Work out the finished part from the listing and answer in its coordinate system (mm). A direction names the side the tool comes from. Round coordinates to 2 decimals unless told otherwise and drop trailing zeros. Write each loop counter-clockwise with the first axis right and the second up, starting at its lowest first coordinate (ties: lowest second). Pieces come first, ordered by that corner, then holes. Notation, with made-up numbers: M 85,2 L 144,2 A14 ccw 144,14 Z; hole C 34.5,63.25 d4. An arc over 180 degrees is marked long. One line per item, written item: value. Start each with the question number.
Q1. A tool of negligible diameter and unlimited length cuts with its end or side. For faces 1 (the flat face through (19.2, -4.8, -2)), 2 (the flat face through (-0.29, -8, 2)), 3 (the flat face through (29.71, -7, 2)), 4 (the flat face through (15, 0, 2)), 5 (the flat face through (15, -15, 2)), from which of +Z, -Z, +X, -X, +Y, -Y can it reach the whole face along a straight path? Write none if from no direction.
Q2. Find section D-D (y = 1.25). Write down the section's boundary in (x, z).
Q3. Find section A-A (y = -7.5). Write down the section's boundary in (x, z).
Q4. Consider probe 1 along Z at (x, y) = (27.5, -16.5); probe 2 along Z at (x, y) = (13, -14); probe 3 along X at (y, z) = (-9.25, -13.5). Determine where each line is inside the solid, lowest interval first.
Q5. Find section B-B (x = 3.5). Write down the section's boundary in (y, z).
Q6. Given pin 1 Ø10 at (x, z) = (7, -12) entering from -Y; pin 2 Ø1 at (x, z) = (19.5, 2) entering from +Y; pin 3 Ø2 at (y, z) = (-7.5, -12) entering from -X; pin 4 Ø10 at (y, z) = (-3, 0.5) entering from +X, each flat-ended and moving along its own axis, determine where each tip first touches the part or whether it passes through.
Q7. Find section C-C (z = -7.25). Write down the section's boundary in (x, y), and give its area (3 significant figures).
Autodesk Inventor part; units mm, degrees
ref_plane "YZ Plane" through (0, 0, 0) normal (1, 0, 0) x (0, 1, 0)
ref_plane "XZ Plane" through (0, 0, 0) normal (0, 1, 0) x (-1, 0, 0)
ref_plane "XY Plane" through (0, 0, 0) normal (0, 0, 1) x (1, 0, 0)
sketch "Boceto1" plane through (0, 0, 0) normal (0, 0, 1) x (1, 0, 0)
  line L0 (-0.2897, 0) -> (29.7103, 0)
  line L1 (29.7103, 0) -> (29.7103, -15)
  line L2 (29.7103, -15) -> (-0.2897, -15)
  line L3 (-0.2897, -15) -> (-0.2897, 0)
  point P0 (0, 0)
  dimension "d0" = 30
  dimension "d1" = 15
extrude "Extrusión1" add sketch "Boceto1" along normal blind 3.3
sketch "Boceto2" plane through (0, 0, 0) normal (0, 0, -1) x (-1, 0, 0)
  line L0 (-29.7103, -15) -> (0.2897, -15)
  line L1 (0.2897, 0) -> (-29.7103, 0)
  line L2 (-29.7103, 0) -> (-29.7103, -15)
  line L3 (-29.7103, -15) -> (0.2897, -15)
  line L4 (0.2897, -15) -> (0.2897, 0)
  line L5 (4.2897, 4) -> (-33.7103, 4)
  line L6 (-33.7103, 4) -> (-33.7103, -19)
  line L7 (-33.7103, -19) -> (4.2897, -19)
  line L8 (4.2897, -19) -> (4.2897, 4)
  point P0 (0, 0)
  dimension "d4" = 4
extrude "Extrusión2" add sketch "Boceto2" along normal blind 2 contours L2 L1 L4 L0 | L8 L7 L6 L5
sketch "Boceto3" plane through (0, 0, -2) normal (0, 0, -1) x (-1, 0, 0)
  line L0 (4.2897, 4) -> (-33.7103, 4)
  line L1 (-14.7103, 4) -> (-14.7103, -19)
  line L2 (-33.7103, -19) -> (4.2897, -19)
  circle A0 centre (-14.7103, -7.5) radius 5
  point P0 (0, 0)
  dimension "d7" = 10
extrude "Extrusión3" add sketch "Boceto3" along normal blind 13
properties part number "boton2"
The answers:
1. face 1: -Z
1. face 2: +Z, -X, +Y, -Y
1. face 3: +Z, +X, +Y, -Y
1. face 4: +Z, +X, -X, +Y
1. face 5: +Z, +X, -X, -Y
2. outline: M -4.29,-2 L 33.71,-2 L 33.71,0 L -4.29,0 Z
3. outline: M -4.29,-2 L 9.71,-2 L 9.71,-15 L 19.71,-15 L 19.71,-2 L 33.71,-2 L 33.71,0 L 29.71,0 L 29.71,3.3 L -0.29,3.3 L -0.29,0 L -4.29,0 Z
4. probe 1: -2 to 0
4. probe 2: -2 to 3.3
4. probe 3: 10.03 to 19.39
5. outline: M -19,-2 L 4,-2 L 4,0 L 0,0 L 0,3.3 L -15,3.3 L -15,0 L -19,0 Z
6. pin 1: y = -11.7
6. pin 2: y = 0
6. pin 3: x = 9.71
6. pin 4: x = 33.71
7. outline: C 14.71,-7.5 d10
7. area: 78.5 mm2
